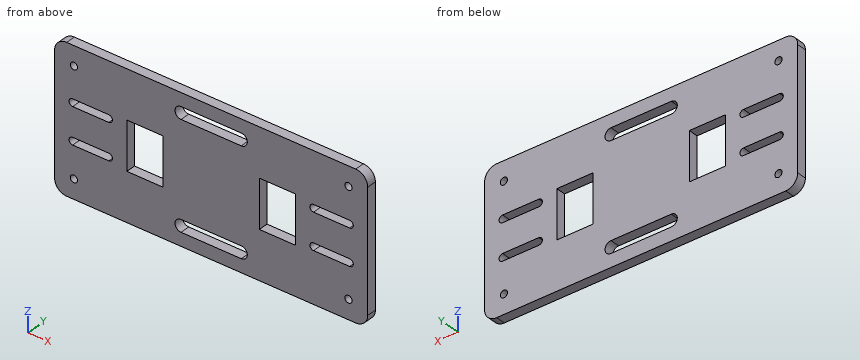
Autodesk Inventor part; units mm, degrees
ref_plane "Mid Plane" through (-61, 26.5, 30) normal (-1, 0, 0) x (0, 0, 1)
ref_plane "YZ Plane" through (0, 0, 0) normal (1, 0, 0) x (0, 1, 0)
ref_plane "XZ Plane" through (0, 0, 0) normal (0, 1, 0) x (-1, 0, 0)
sketch "Motor Support" plane through (0, 0, 0) normal (1, 0, 0) x (0, 1, 0)
  circle A0 centre (0, 0) radius 11.25
  line L0 (-12.5, -22.5) -> (22.5, -22.5)
  line L1 (22.5, -22.5) -> (22.5, 22.5)
  line L2 (22.5, 22.5) -> (-12.5, 22.5)
  line L3 (-22.5, 12.5) -> (-22.5, -12.5)
  arc A1 (-12.5, 22.5) -> (-22.5, 12.5) centre (-12.5, 12.5) ccw
  arc A2 (-22.5, -12.5) -> (-12.5, -22.5) centre (-12.5, -12.5) ccw
  circle A3 centre (15.5, 15.5) radius 1.5
  circle A4 centre (15.5, -15.5) radius 1.5
  circle A5 centre (-15.5, 15.5) radius 1.5
  circle A6 centre (-15.5, -15.5) radius 1.5
  point P0 (-22.5, 22.5)
  point P1 (22.5, 0)
  dimension "d0" = 22.5
  dimension "d1" = 45
  dimension "d2" = 45
  dimension "d3" = 10
  dimension "d4" = 22.5
  dimension "d5" = 3
  dimension "d6" = 3
  dimension "d7" = 3
  dimension "d8" = 3
  dimension "d9" = 31
  dimension "d10" = 31
  dimension "d11" = 15.5
  dimension "d12" = 15.5
extrude "Motor Support E" add sketch "Motor Support" along normal blind 4
sketch "Base" plane through (0, 22.5, 22.5) normal (0, 1, 0) x (1, 0, 0)
  line L0 (0, 45) -> (0, 0)
  line L1 (0, 0) -> (4, 0)
  line L2 (4, 45) -> (4, 0)
  line L3 (0, 45) -> (4, 45)
  line L4 (4, -7.5) -> (-61, -7.5)
  line L5 (-61, -7.5) -> (-61, 52.5)
  line L6 (-61, 52.5) -> (4, 52.5)
  line L7 (4, 52.5) -> (4, -7.5)
  line L8 (-41, 32.5) -> (-26, 32.5)
  line L9 (-26, 32.5) -> (-26, 12.5)
  line L10 (-26, 12.5) -> (-41, 12.5)
  line L11 (-41, 12.5) -> (-41, 32.5)
  point P0 (0, 22.5)
  point P1 (4, 22.5)
  point P2 (-26, 22.5)
  point P3 (0, 22.5)
  dimension "d15" = 65
  dimension "d16" = 60
  dimension "d19" = 15
  dimension "d20" = 20
  dimension "d21" = 26
extrude "Base E" add sketch "Base" along normal blind 4
ref_plane "Mid Plane" through (-61, 26.5, 30) normal (-1, 0, 0) x (0, 0, 1)
mirror "Mirror Base" about plane through (-61, 26.5, 30) normal (-1, 0, 0)
fillet "Fillet1" radius 5 4 edges at (4, 24.5, 30) (4, 24.5, -30) (-126, 24.5, 30) (-126, 24.5, -30)
fillet "Fillet2" radius 5 4 edges at (2, 22.5, -22.5) (2, 22.5, 22.5) (-124, 22.5, -22.5) (-124, 22.5, 22.5)
sketch "Base Hole Pattern" plane through (0, 26.5, 22.5) normal (0, 1, 0) x (1, 0, 0)
  circle A0 centre (-4, 0.5) radius 1.5
  circle A1 centre (-118, 44.5) radius 1.5
  circle A2 centre (-118, 0.5) radius 1.5
  circle A3 centre (-4, 44.5) radius 1.5
  arc A4 (-121, 52.5) -> (-126, 47.5) centre (-121, 47.5) ccw
  line L0 (-126, -2.5) -> (-126, 47.5)
  arc A5 (-126, -2.5) -> (-121, -7.5) centre (-121, -2.5) ccw
  line L1 (-1, -7.5) -> (-121, -7.5)
  arc A6 (-1, -7.5) -> (4, -2.5) centre (-1, -2.5) ccw
  line L2 (4, -2.5) -> (4, 47.5)
  arc A7 (4, 47.5) -> (-1, 52.5) centre (-1, 47.5) ccw
  line L3 (-1, 52.5) -> (-121, 52.5)
  line L4 (-81, 32.5) -> (-96, 32.5)
  line L5 (-81, 12.5) -> (-81, 32.5)
  line L6 (-96, 12.5) -> (-81, 12.5)
  line L7 (-96, 32.5) -> (-96, 12.5)
  line L8 (-41, 32.5) -> (-26, 32.5)
  line L9 (-26, 32.5) -> (-26, 12.5)
  line L10 (-26, 12.5) -> (-41, 12.5)
  line L11 (-41, 12.5) -> (-41, 32.5)
  line L12 (-73.5, 44.5) -> (-48.5, 44.5) construction
  line L13 (-73.5, 42) -> (-48.5, 42)
  line L14 (-48.5, 47) -> (-73.5, 47)
  arc A8 (-73.5, 47) -> (-73.5, 42) centre (-73.5, 44.5) ccw
  arc A9 (-48.5, 42) -> (-48.5, 47) centre (-48.5, 44.5) ccw
  line L15 (-73.5, 0.5) -> (-48.5, 0.5) construction
  line L16 (-73.5, -2) -> (-48.5, -2)
  line L17 (-48.5, 3) -> (-73.5, 3)
  arc A10 (-73.5, 3) -> (-73.5, -2) centre (-73.5, 0.5) ccw
  arc A11 (-48.5, -2) -> (-48.5, 3) centre (-48.5, 0.5) ccw
  line L18 (-118.5, 30) -> (-103.5, 30) construction
  line L19 (-118.5, 28.5) -> (-103.5, 28.5)
  line L20 (-103.5, 31.5) -> (-118.5, 31.5)
  arc A12 (-118.5, 31.5) -> (-118.5, 28.5) centre (-118.5, 30) ccw
  arc A13 (-103.5, 28.5) -> (-103.5, 31.5) centre (-103.5, 30) ccw
  line L21 (-118.5, 15) -> (-103.5, 15) construction
  line L22 (-118.5, 13.5) -> (-103.5, 13.5)
  line L23 (-103.5, 16.5) -> (-118.5, 16.5)
  arc A14 (-118.5, 16.5) -> (-118.5, 13.5) centre (-118.5, 15) ccw
  arc A15 (-103.5, 13.5) -> (-103.5, 16.5) centre (-103.5, 15) ccw
  line L24 (-18.5, 30) -> (-3.5, 30) construction
  line L25 (-18.5, 28.5) -> (-3.5, 28.5)
  line L26 (-3.5, 31.5) -> (-18.5, 31.5)
  arc A16 (-18.5, 31.5) -> (-18.5, 28.5) centre (-18.5, 30) ccw
  arc A17 (-3.5, 28.5) -> (-3.5, 31.5) centre (-3.5, 30) ccw
  line L27 (-18.5, 15) -> (-3.5, 15) construction
  line L28 (-18.5, 13.5) -> (-3.5, 13.5)
  line L29 (-3.5, 16.5) -> (-18.5, 16.5)
  arc A18 (-18.5, 16.5) -> (-18.5, 13.5) centre (-18.5, 15) ccw
  arc A19 (-3.5, 13.5) -> (-3.5, 16.5) centre (-3.5, 15) ccw
  point P0 (-61, 44.5)
  point P1 (-61, 52.5)
  point P2 (-61, 0.5)
  point P3 (-111, 30)
  point P4 (-111, 15)
  point P5 (-11, 30)
  point P6 (-11, 15)
  dimension "d29" = 3
  dimension "d30" = 3
  dimension "d33" = 3
  dimension "d34" = 3
  dimension "d35" = 8
  dimension "d36" = 8
  dimension "d37" = 8
  dimension "d38" = 8
  dimension "d43" = 25
  dimension "d44" = 5
  dimension "d45" = 25
  dimension "d46" = 2.5
  dimension "d47" = 15
  dimension "d48" = 3
  dimension "d49" = 15
  dimension "d50" = 3
  dimension "d51" = 15
  dimension "d52" = 15
  dimension "d53" = 22.5
  dimension "d56" = 15
  dimension "d57" = 3
  dimension "d58" = 15
  dimension "d59" = 3
  dimension "d60" = 15
  dimension "d61" = 22.5
  dimension "d62" = 15
extrude "Spacer Holes" cut sketch "Base Hole Pattern" against normal blind 10 contours A0 | A1 | A2 | A3
extrude "Base Slots" cut sketch "Base Hole Pattern" against normal blind 10 contours A8 L14 A9 L13 | A10 L17 A11 L16 | A12 L20 A13 L19 | A14 L23 A15 L22 | A16 L26 A17 L25 | A18 L29 A19 L28
sketch "Sketch6" plane through (-122, -22.5, -12.5) normal (0, -1, 0) x (1, 0, 0)
  line L0 (-11.238, 55.4401) -> (134.3481, 55.4401)
  line L1 (134.3481, 55.4401) -> (134.3481, -24.4895)
  line L2 (134.3481, -24.4895) -> (-11.238, -24.4895)
  line L3 (-11.238, -24.4895) -> (-11.238, 55.4401)
  point P0 (122, 12.5)
extrude "Extrusion7" cut sketch "Sketch6" against normal up to surface (45 mm away)
equation "\"d6\" = d5"
equation "\"d7\" = d5"
equation "\"d8\" = d5"
equation "\"d30\" = d29"
equation "\"d33\" = d29"
equation "\"d34\" = d29"
equation "\"d36\" = d35"
equation "\"d37\" = d35"
equation "\"d38\" = d35"
equation "\"d45\" = d43"
equation "\"d46\" = 0.5 * d44"
equation "\"d49\" = d47"
equation "\"d50\" = d48"
equation "\"d56\" = d47"
equation "\"d57\" = d48"
equation "\"d58\" = d47"
equation "\"d59\" = d48"
properties part number "Top"
Part model, mm, in its own coordinate system. Coordinates: 2 decimals unless noted, no trailing zeros. Loops run counter-clockwise (first coordinate to the right, second up) from the corner with the lowest first, then second, coordinate; pieces in that order, holes last. Notation, with made-up numbers: (-22, 87.5) - (30, 87.5) arc R16 cw to (30, 117.5) - close; hole circle Ø2 at (72.5, 10.5). An arc over 180 degrees is marked (long way). Write each question's results on one line, items separated by ' | '. Start each with the question number.
Q1. Probe line 1 along Z through (x, y) = (-52.5, 24.85); line 2 along X through (y, z) = (25.75, 22); line 3 along X through (y, z) = (24.15, 0). List the from-to ranges inside material, lowest first.
Q2. Slice it at D-D on y = 23.15. Give the number of separate pieces and of enclosed holes in the cut face, and give its area (3 significant figures).
Q3. Slice it at A-A on x = -38. Give the cut face in (y, z), and give its area (3 significant figures).
Q4. Slice it at B-B on z = -22. Give the cut face in (x, y).
Q5. Slice it at C-C on z = -7.5. Give the cut face in (x, y), and give its area (3 significant figures).
Q6. Drop a flat-ended pin along its axis: pin 1 Ø2.5 at (x, z) = (-118, -22) entering from -Y. Give the stop position or say it passes through.
Answer:
1) line 1: z = -30 to -24.5, -19.5 to 19.5, 24.5 to 30 | line 2: x = -126 to -119.5, -116.5 to -76, -46 to -5.5, -2.5 to 4 | line 3: x = -126 to -96, -81 to -41, -26 to 4
2) separate pieces: 1 | enclosed holes: 12 | area: 6,650 mm2
3) outline: (22.5, -30) - (26.5, -30) - (26.5, -10) - (22.5, -10) - close; (22.5, 10) - (26.5, 10) - (26.5, 30) - (22.5, 30) - close | area: 160 mm2
4) outline: (-126, 22.5) - (-119.5, 22.5) - (-119.5, 26.5) - (-126, 26.5) - close; (-116.5, 22.5) - (-76, 22.5) - (-76, 26.5) - (-116.5, 26.5) - close; (-46, 22.5) - (-5.5, 22.5) - (-5.5, 26.5) - (-46, 26.5) - close; (-2.5, 22.5) - (4, 22.5) - (4, 26.5) - (-2.5, 26.5) - close
5) outline: (-126, 22.5) - (-120, 22.5) - (-120, 26.5) - (-126, 26.5) - close; (-102, 22.5) - (-96, 22.5) - (-96, 26.5) - (-102, 26.5) - close; (-81, 22.5) - (-41, 22.5) - (-41, 26.5) - (-81, 26.5) - close; (-26, 22.5) - (-20, 22.5) - (-20, 26.5) - (-26, 26.5) - close; (-2, 22.5) - (4, 22.5) - (4, 26.5) - (-2, 26.5) - close | area: 256 mm2
6) pin 1: passes through
